Source: three-view drawing plus pictorial views. Frame: mm from the lowest corner of the part. A direction names the side the tool comes from. Round coordinates to 2 decimals unless told otherwise and drop trailing zeros. Order: outer loops, then holes, each group sorted by start corner. A loop starts at its lowest first (then second) coordinate and runs counter-clockwise, first axis right, second up. Notation, with made-up numbers: M 8.25,80 L 16.25,80 A35 ccw 16.25,116 Z; hole C 62.5,24 d11. An arc over 180 degrees is marked long. Return JSON: item names as keys, results as strings. Group by question number.
Q1. Cut plane B-B on x = 14. Output: boundary loops of the cut face in (y, z).
Q2. Contact query for flat-ended pins moving along their axis: pin 1 (3.5 mm diameter, centred on y = 12.7, z = 8.3, fed in from +X); pin 2 (3 mm diameter, centred on x = 19, z = 5, fed in from -Y); pin 3 (2.5 mm diameter, centred on y = 62.3, z = 18.3, fed in from +X); pin 4 (2.5 mm diameter, centred on y = 11, z = 17.5, fed in from -X). Output: stop coordinate, or through.
Q3. Access query for the marked faces 1, 2 and 3. Directions: +Z, -Z, +X, -X, +Y, -Y. A direction counts if a zero-diameter tool reaches every point of the face in a straight line with its end or side. Return the directions, or none.
Q4. Ray query, probe 1 along Y at (x, z) = (16.65, 8.3); probe 2 along X at (y, z) = (70, 1.7); probe 3 along Y at (x, z) = (41, 2). Return the intervals inside material, ascending.
Q5. Cut plane C-C on y = 12.7. Output: boundary loops of the cut face in (x, z), and give its area (4 significant figures).
Q6. Cut plane A-A on z = 18.3. Output: boundary loops of the cut face in (x, y).
Q7. Cut plane D-D on z = 21.75. Output: boundary loops of the cut face in (x, y).
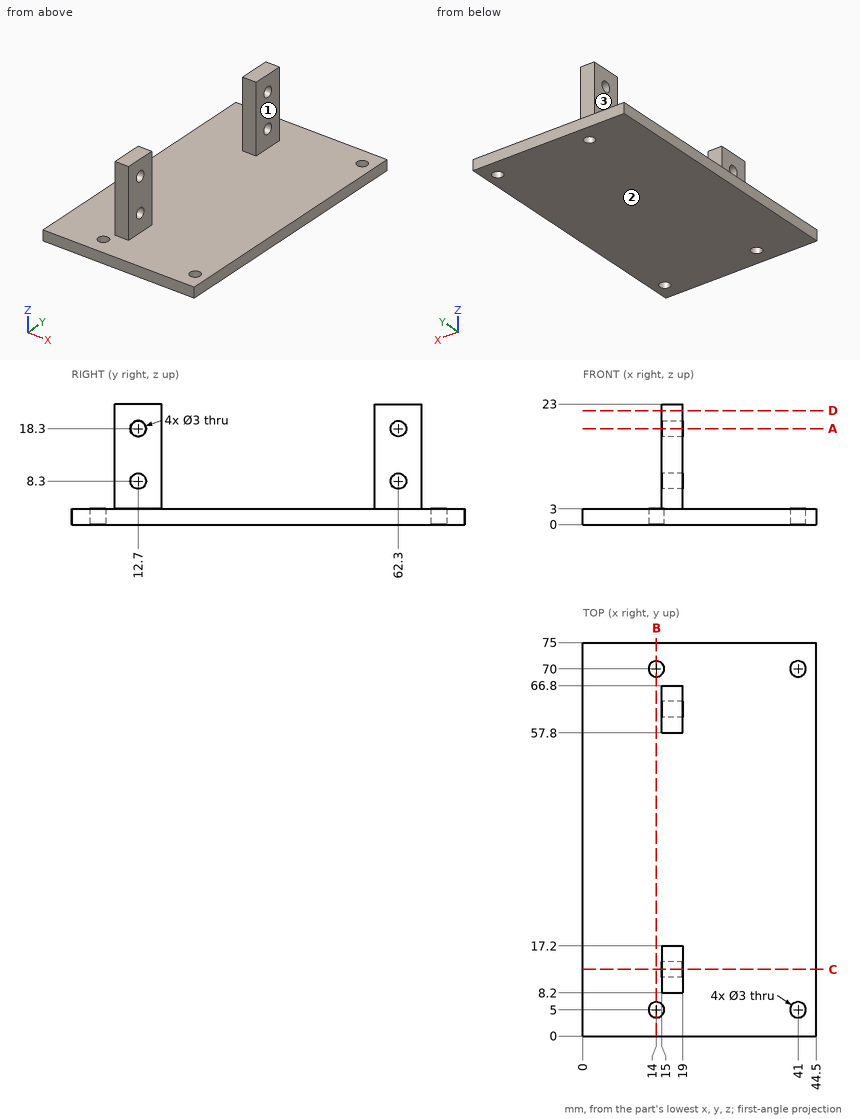
Result sheet:
{
 "1": {"outline": "M 0,0 L 3.5,0 L 3.5,3 L 0,3 Z; M 6.5,0 L 68.5,0 L 68.5,3 L 6.5,3 Z; M 71.5,0 L 75,0 L 75,3 L 71.5,3 Z"},
 "2": {"pin 1": "stops at x = 19", "pin 2": "stops at y = 8.2", "pin 3": "passes through", "pin 4": "stops at x = 15"},
 "3": {"face 1": "+Z, +X, +Y, -Y", "face 2": "-Z, +X, -X, +Y, -Y", "face 3": "+Z, -X, +Y, -Y"},
 "4": {"probe 1": "y = 8.2 to 11.2, 14.2 to 17.2, 57.8 to 60.8, 63.8 to 66.8", "probe 2": "x = 0 to 12.5, 15.5 to 39.5, 42.5 to 44.5", "probe 3": "y = 0 to 3.5, 6.5 to 68.5, 71.5 to 75"},
 "5": {"outline": "M 0,0 L 44.5,0 L 44.5,3 L 19,3 L 19,6.8 L 15,6.8 L 15,3 L 0,3 Z; M 15,9.8 L 19,9.8 L 19,16.8 L 15,16.8 Z; M 15,19.8 L 19,19.8 L 19,23 L 15,23 Z", "area": "189.5 mm²"},
 "6": {"outline": "M 15,8.2 L 19,8.2 L 19,11.2 L 15,11.2 Z; M 15,14.2 L 19,14.2 L 19,17.2 L 15,17.2 Z; M 15,57.8 L 19,57.8 L 19,60.8 L 15,60.8 Z; M 15,63.8 L 19,63.8 L 19,66.8 L 15,66.8 Z"},
 "7": {"outline": "M 15,8.2 L 19,8.2 L 19,17.2 L 15,17.2 Z; M 15,57.8 L 19,57.8 L 19,66.8 L 15,66.8 Z"}
}
